```python
from build123d import *

# Parameters (mm, degrees)
SKETCH2_W           = 12
SKETCH2_H           = 22.9
BOSS_EXTRUDE1_DEPTH = 22.6
SKETCH3_W           = 12
SKETCH3_H           = 2.5
BOSS_EXTRUDE2_DEPTH = 32.2
BOSS_EXTRUDE3_DEPTH = 4
SKETCH7_R           = 2.3
BOSS_EXTRUDE4_DEPTH = 3
CUT_EXTRUDE1_DEPTH  = 2.5
SKETCH10_R          = 0.85
CUT_EXTRUDE2_DEPTH  = 2.5
SKETCH12_W          = 3.6
SKETCH12_H          = 1.2
BOSS_EXTRUDE5_DEPTH = 10.5


with BuildPart() as part:
    # Sketch2 → Boss-Extrude1 (new body)
    with BuildSketch(Plane(origin=(0, 0, 0), x_dir=(1, 0, 0), z_dir=(0, 1, 0))):
        with Locations((6, 11.45)):
            Rectangle(SKETCH2_W, SKETCH2_H)
    extrude(amount=BOSS_EXTRUDE1_DEPTH)

    # Sketch3 → Boss-Extrude2 (add)
    with BuildSketch(Plane.XY.offset(4.7)):
        with Locations((6, 17.15)):
            Rectangle(SKETCH3_W, SKETCH3_H)
    extrude(amount=-BOSS_EXTRUDE2_DEPTH)

    # Sketch5 → Boss-Extrude3 (add)
    with BuildSketch(Plane(origin=(0, 22.6, 0), x_dir=(1, 0, 0), z_dir=(0, 1, 0))):
        with BuildLine():
            Line((3.515017185, 12.299982102), (3.515017185, 11.461214188))
            ThreePointArc((3.515017185, 11.461214188), (5.98348051, 2.2741e-05), (8.515017185, 11.447447894))
            Line((8.515017185, 11.447447894), (8.515017185, 12.299982102))
            ThreePointArc((8.515017185, 12.299982102), (6.015017185, 14.799982102), (3.515017185, 12.299982102))
        make_face()
    extrude(amount=BOSS_EXTRUDE3_DEPTH)

    # Sketch7 → Boss-Extrude4 (add)
    with BuildSketch(Plane(origin=(0, 26.6, 0), x_dir=(1, 0, 0), z_dir=(0, 1, 0))):
        with Locations(Location((5.9, 5.9, 0), (0, 0, 270))):
            Circle(SKETCH7_R)
    extrude(amount=BOSS_EXTRUDE4_DEPTH)

    # Sketch9 → Cut-Extrude1 (cut)
    with BuildSketch(Plane(origin=(0, 18.4, 0), x_dir=(1, 0, 0), z_dir=(0, 1, 0))):
        with BuildLine():
            Line((5.35, 27.5), (6.65, 27.5))
            Line((6.65, 27.5), (6.65, 26.148683298))
            ThreePointArc((6.65, 26.148683298), (6, 24.05), (5.35, 26.148683298))
            Line((5.35, 26.148683298), (5.35, 27.5))
        make_face()
        with BuildLine():
            Line((6.75, -4.7), (6.65, -3.248683298))
            ThreePointArc((6.65, -3.248683298), (6, -1.15), (5.35, -3.248683298))
            Line((5.35, -3.248683298), (5.45, -4.7))
            Line((5.45, -4.7), (6.75, -4.7))
        make_face()
    extrude(amount=-CUT_EXTRUDE1_DEPTH, mode=Mode.SUBTRACT)

    # Sketch10 → Cut-Extrude2 (cut)
    with BuildSketch(Plane(origin=(0, 29.6, 0), x_dir=(1, 0, 0), z_dir=(0, 1, 0))):
        with Locations(Location((5.87814142, 5.916228473, 0), (0, 0, 270))):
            Circle(SKETCH10_R)
    extrude(amount=-CUT_EXTRUDE2_DEPTH, mode=Mode.SUBTRACT)

    # Sketch12 → Boss-Extrude5 (add)
    with BuildSketch(Plane.XY):
        with Locations((6, 4.377974725)):
            Rectangle(SKETCH12_W, SKETCH12_H)
    extrude(amount=BOSS_EXTRUDE5_DEPTH)


solid = part.part
```
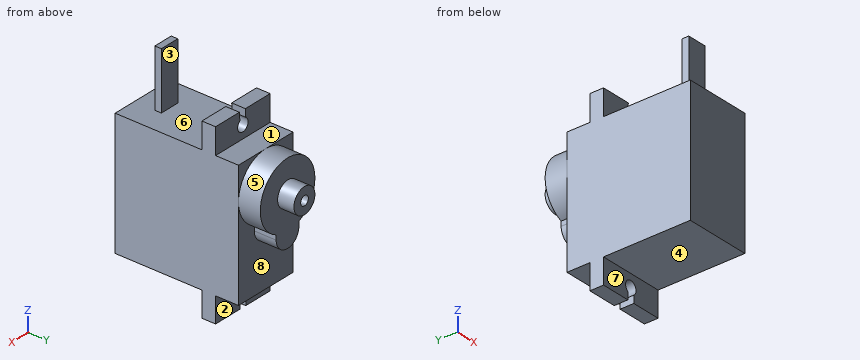
CAD build for the part. Positions are in the model's coordinates, mm. Face numbers are marked on the shaded views. A direction names the side the tool comes from. Round coordinates to 2 decimals unless told otherwise and drop trailing zeros. Loops run counter-clockwise (first coordinate to the right, second up) from the corner with the lowest first, then second, coordinate; pieces in that order, holes last. Notation, with made-up numbers: M 82.5,-5 L 111.5,-5 A19 ccw 111.5,2 Z; hole C 33,-4.5 d2. An arc over 180 degrees is marked long. Return JSON: item names as keys, results as strings. Group by question number.
(1) Tool access for the marked faces 1, 2, 3, 4 and 5: list every direction of +Z, -Z, +X, -X, +Y, -Y with a clear straight run to the whole face (end or side of a thin tool).
(2) Mould opens along Y. For the marked faces 6, 7 and 8 say: +Y half, -Y half, draft (parallel to the pull), parting line (faces both ways), or undercut.
(3) Saw through at D-D, the plane y = 23. List the corners of the cut face in (x, z), and give its area (3 significant figures).
(4) Wall check: probe 1 along X at (y, z) = (16.95, -25.2); probe 2 along Y at (x, z) = (5.25, -18.5); probe 3 along Y at (x, z) = (8.75, -26). Give the ranges that are in metal, low to high. Write a range as [from, to].
(5) Saw through at B-B, the plane z = -25.2. List the corners of the cut face in (x, y), and give its area (4 significant figures).
(6) Saw through at A-A, the plane z = 2.3. List the corners of the cut face in (x, y).
(7) Drop flat-ended pins along their axis: P1, Ø1.1, axis at x = 5, z = 7.5, coming from the +Y side; P2, Ø1, axis at y = 4.5, z = 6, coming from the +X side; P3, Ø2.5, axis at x = 4, z = -25, coming from the +Y side. Give the stop position or say it passes through.
(8) Saw through at C-C, the plane x = 9.5. List the corners of the cut face in (y, z), and give its area (3 significant figures).
Answer list:
{
 "1": {"face 1": "+Z, +X, -X, +Y", "face 2": "-Z, +X, -X, +Y", "face 3": "+Z, +X, -X", "face 4": "-Z, +X, -X, -Y", "face 5": "+Y"},
 "2": {"face 6": "undercut", "face 7": "-Y half", "face 8": "+Y half"},
 "3": {"outline": "M 3.52,-12.3 A2.5 ccw 8.52,-12.3 L 8.52,-11.45 A6 ccw long 3.52,-11.46 Z", "area": "125 mm2"},
 "4": {"probe 1": "[0, 4.85], [7.15, 12]", "probe 2": "[0, 22.6]", "probe 3": "[15.9, 18.4]"},
 "5": {"outline": "M 0,15.9 L 4.85,15.9 L 4.85,18.4 L 0,18.4 Z; M 7.15,15.9 L 12,15.9 L 12,18.4 L 7.15,18.4 Z", "area": "24.25 mm2"},
 "6": {"outline": "M 0,15.9 L 4.85,15.9 L 4.85,18.4 L 0,18.4 Z; M 4.2,3.78 L 7.8,3.78 L 7.8,4.98 L 4.2,4.98 Z; M 7.15,15.9 L 12,15.9 L 12,18.4 L 7.15,18.4 Z"},
 "7": {"P1": "y = 4.98", "P2": "x = 7.8", "P3": "y = 18.4"},
 "8": {"outline": "M 0,-22.9 L 15.9,-22.9 L 15.9,-27.5 L 18.4,-27.5 L 18.4,-22.9 L 22.6,-22.9 L 22.6,-10.87 L 26.6,-10.87 L 26.6,-1.13 L 22.6,-1.13 L 22.6,0 L 18.4,0 L 18.4,4.7 L 15.9,4.7 L 15.9,0 L 0,0 Z", "area": "580 mm2"}
}
